from build123d import *

# Parameters (mm, degrees)
CROQUIS2_W              = 0.5
CROQUIS2_H              = 0.5
SALIENTE_EXTRUIR1_DEPTH = 13.5


with BuildPart() as part:
    # Croquis1 → Revolución1 (revolve)
    with BuildSketch(Plane.XY):
        with BuildLine():
            Line((0, 0), (2.299223692, 0))
            Line((2.299223692, 0), (2.299223692, 7.084178562))
            ThreePointArc((2.299223692, 7.084178562), (1.350090731, 8.117657033), (0, 8.5))
            Line((0, 8.5), (0, 0))
        make_face()
    revolve(axis=Axis((0, 8.5, 0), (0, -1, 0)))

    # Croquis2 → Saliente-Extruir1 (add)
    with BuildSketch(Plane.XZ):
        with Locations((1.27, 0)):
            Rectangle(CROQUIS2_W, CROQUIS2_H)
        with Locations((-1.27, 0)):
            Rectangle(CROQUIS2_W, CROQUIS2_H)
    extrude(amount=SALIENTE_EXTRUIR1_DEPTH)


solid = part.part
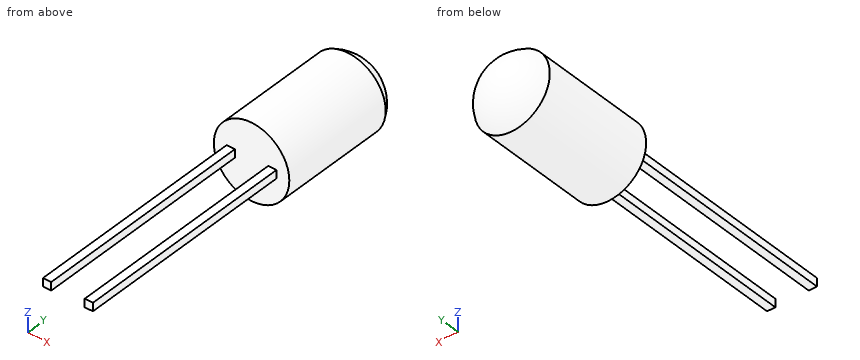
Source: CAD feature listing. Evaluate the final solid. Frame: model axes, mm. Round coordinates to 2 decimals unless told otherwise and drop trailing zeros. Order: outer loops, then holes, each group sorted by start corner. A loop starts at its lowest first (then second) coordinate and runs counter-clockwise, first axis right, second up. Notation, with made-up numbers: (31.25, 15.5) - (55.25, 15.5) arc R22 cw to (55.25, 40.5) - close; hole circle Ø6 at (0.5, -5). An arc over 180 degrees is marked (long way). Use a Markdown table: item, result. Add a question column.
1. First-contact query: pin 1 (1.5 mm diameter, centred on x = -0.5, z = 0, fed in from -Y); pin 2 (1 mm diameter, centred on x = 1.5, y = 1, fed in from -Z); pin 3 (0.6 mm diameter, centred on x = -1, y = -7.5, fed in from -Z). Flat tips, straight axial feed; report the tip coordinate or a pass-through.
2. Section query C-C (x = 0). Return the cut outline in (y, z), then the cut area to 3 significant figures.
3. Section query A-A (y = -7). Return the cut outline in (x, z).
4. Section query B-B (z = 0). Return the cut outline in (x, y), then the cut area to 3 significant figures.
5. Line query: probe 1 along X at (y, z) = (-8.75, 0.05); probe 2 along Z at (x, y) = (1.15, -9.5); probe 3 along Y at (x, z) = (-0.6, -0.3). Output: solid intervals per line, ascending.
6. Section query D-D (y = 1.75). Return the cut outline in (x, z), then the cut area to 3 significant figures.
Derived:
| question | item | result |
|---|---|---|
| 1 | pin 1 | y = -13.5 |
| 1 | pin 2 | z = -2.07 |
| 1 | pin 3 | z = -0.25 |
| 2 | outline | (0, -2.3) - (7.08, -2.3) arc R2.57 ccw to (7.08, 2.3) - (0, 2.3) - close |
| 2 | area | 37.2 mm2 |
| 3 | outline | (-1.52, -0.25) - (-1.02, -0.25) - (-1.02, 0.25) - (-1.52, 0.25) - close; (1.02, -0.25) - (1.52, -0.25) - (1.52, 0.25) - (1.02, 0.25) - close |
| 4 | outline | (-2.3, 0) - (-1.52, 0) - (-1.52, -13.5) - (-1.02, -13.5) - (-1.02, 0) - (1.02, 0) - (1.02, -13.5) - (1.52, -13.5) - (1.52, 0) - (2.3, 0) - (2.3, 7.08) arc R2.57 ccw to (-2.3, 7.08) - close |
| 4 | area | 50.7 mm2 |
| 5 | probe 1 | -1.52 to -1.02, 1.02 to 1.52 |
| 5 | probe 2 | -0.25 to 0.25 |
| 5 | probe 3 | 0 to 8.41 |
| 6 | outline | circle Ø4.6 at (0, 0) |
| 6 | area | 16.6 mm2 |
